```python
from build123d import *

# Parameters (mm, degrees)
F0_W     = 76.2
F0_H     = 55.5625
F1_DEPTH = 25.4
F2_R     = 55.56249
F3_R     = 9.525
F4_DEPTH = 25.4
F6_DEPTH = 55.5635


# Not quite as in the source:
# - a fillet or chamfer is up to 0.001 mm smaller than in the source, because OpenCascade refuses the exact size


with BuildPart() as f1:
    # F0 (on Right) → F1 (new body)
    with BuildSketch(Plane.YZ):
        Rectangle(F0_W, F0_H)
    extrude(amount=F1_DEPTH)

    # F2 (radius 55.5625 in the source; OpenCascade refuses exactly that, so slightly less here)
    f2_edges = [f1.edges().sort_by_distance(p)[0] for p in [
        (12.7, 38.1, -27.78125),
    ]]
    fillet(f2_edges, radius=F2_R)

    # F3 (on face) → F4 (cut)
    with BuildSketch(Plane.YZ.offset(25.4)):
        with Locations((10.31875, 0)):
            Circle(F3_R)
    extrude(amount=-F4_DEPTH, mode=Mode.SUBTRACT)

    # F5 (on face) → F6 (cut, through all)
    with BuildSketch(Plane.XY.offset(27.78125)):
        Polygon((0, -38.1), (25.4, -38.1), (0, -12.7), align=None)
    extrude(amount=-F6_DEPTH, mode=Mode.SUBTRACT)


solid = f1.part
```
Read the model definition and answer for the solid it produces. Units are mm, in the model's axes. Coordinates: 2 decimals unless noted, no trailing zeros. Loops run counter-clockwise (first coordinate to the right, second up) from the corner with the lowest first, then second, coordinate; pieces in that order, holes last. Notation, with made-up numbers: (53, 2.25) - (60, 2.25) arc R28 cw to (60, 24.25) - close; hole circle Ø5 at (-2.75, -36.75). An arc over 180 degrees is marked (long way). Answer in a Markdown table with one row per item.
1. Determine the mould class of faces 1 (the face through (12.878, 0.803, 0.419)), 2 (the face through (0, 1, 7)), 3 (the face through (12.88, 21.39, -11.94)) for opening direction Y: +Y half, -Y half, draft (parallel to the pull), parting line (faces both ways), or undercut.
Conclusion:
| item | result |
|---|---|
| face 1 | undercut |
| face 2 | draft |
| face 3 | +Y half |
2. Find section B-B, the plane y = 2. Write down the section's boundary in (x, z).
Conclusion:
| item | result |
|---|---|
| outline | (0, -24.26) - (25.4, -24.26) - (25.4, -4.64) - (0, -4.64) - close; (0, 4.64) - (25.4, 4.64) - (25.4, 27.78) - (0, 27.78) - close |
3. Straight lines are drawn through the part: line 1 (Y direction, x = 13.75, z = -1); line 2 (Z direction, x = 13.75, y = 7); line 3 (Y direction, x = 22.25, z = -5). For each, find the intervals that lie inside material, in ascending order.
Conclusion:
| item | result |
|---|---|
| line 1 | y = -26.45 to 0.85, 19.79 to 30.06 |
| line 2 | z = -22.11 to -8.93, 8.93 to 27.78 |
| line 3 | y = -34.95 to 2.21, 18.43 to 27.4 |
4. Given pin 1 (1.5 mm diameter, centred on x = 16.5, z = -10.5, fed in from +Y); pin 2 (3 mm diameter, centred on y = -24, z = -4.5, fed in from -X), each flat-ended and moving along its own axis, determine where each tip first touches the part or whether it passes through.
Conclusion:
| item | result |
|---|---|
| pin 1 | stops at y = 23.51 |
| pin 2 | stops at x = 9.8 |
5. Find section A-A, the plane z = 7. Write down the section's boundary in (x, y).
Conclusion:
| item | result |
|---|---|
| outline | (0, -12.7) - (25.4, -38.1) - (25.4, 3.86) - (0, 3.86) - close; (0, 16.78) - (25.4, 16.78) - (25.4, 34.07) - (0, 34.07) - close |
6. Find section D-D, the plane y = -30. Write down the section's boundary in (x, z), then the cut area to 3 significant figures.
Conclusion:
| item | result |
|---|---|
| outline | (17.3, -27.78) - (25.4, -27.78) - (25.4, 27.78) - (17.3, 27.78) - close |
| area | 450 mm² |
